Can you work these out from the drawing? Everything is in mm from the part's minimum corner. Coordinates: 2 decimals unless noted, no trailing zeros. Loops run counter-clockwise (first coordinate to the right, second up) from the corner with the lowest first, then second, coordinate; pieces in that order, holes last. Notation, with made-up numbers: (45.25, -37) - (78.25, -37) arc R14 ccw to (78.25, -30) - close; hole circle Ø10 at (36, -22.75). An arc over 180 degrees is marked (long way). Put each result on its own line as item: value. Start each with the question number.
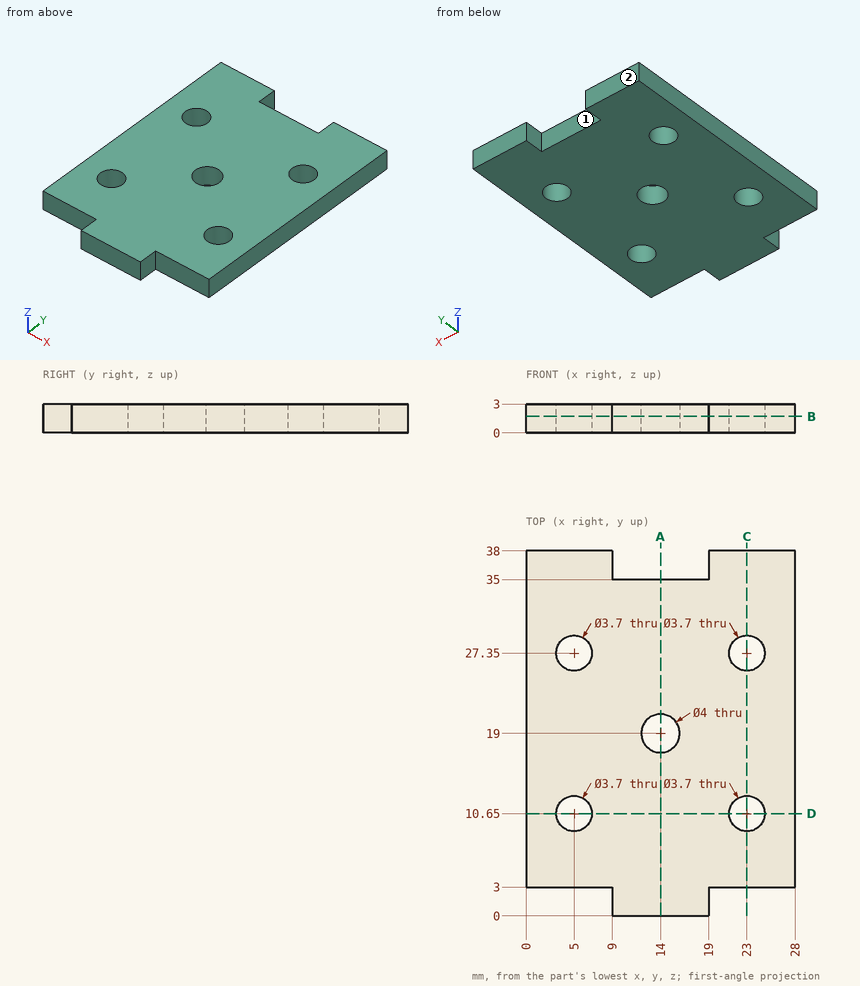
(1) I want a section at B-B on z = 1.7. List the corners of the cut face in (x, y) for me.
(2) I need wall thicknesses on L1, parallel to Y at x = 23, z = 1.85; L2, parallel to X at y = 9.5, z = 2.1; L3, parallel to Y at x = 22, z = 2.8. Which ranges of each line are inside material? Lowest first, please. Write a range as [from, to].
(3) For pin 1 Ø1.5 at (x, z) = (21.5, 1.5) entering from -Y; pin 2 Ø1.5 at (y, z) = (1.5, 1) entering from -X; pin 3 Ø0.9 at (x, z) = (15, 2) entering from +Y, each with a flat end and sliding along its axis, tell me the tip position at first contact or that it passes through.
(4) I want a section at C-C on x = 23. List the corners of the cut face in (y, z) for me.
(5) I want a section at A-A on x = 14. List the corners of the cut face in (y, z) for me, and give its area (3 significant figures).
(6) I want a section at D-D on y = 10.65. List the corners of the cut face in (x, z) for me.
(7) If we mould it in two halves opening along X, with no side actions, what happens to the marked faces 1 and 2? For each: pulls with the +X half, pulls with the -X half, needs draft (parallel to the pull), parting line crosses it, or undercut.
Answer sheet:
1. outline: (0, 3) - (9, 3) - (9, 0) - (19, 0) - (19, 3) - (28, 3) - (28, 38) - (19, 38) - (19, 35) - (9, 35) - (9, 38) - (0, 38) - close; hole circle Ø3.7 at (5, 10.65); hole circle Ø3.7 at (5, 27.35); hole circle Ø4 at (14, 19); hole circle Ø3.7 at (23, 10.65); hole circle Ø3.7 at (23, 27.35)
2. L1: y = [3, 8.8], [12.5, 25.5], [29.2, 38]
2. L2: x = [0, 3.55], [6.45, 21.55], [24.45, 28]
2. L3: y = [3, 9.09], [12.21, 25.79], [28.91, 38]
3. pin 1: stops at y = 3
3. pin 2: stops at x = 9
3. pin 3: stops at y = 35
4. outline: (3, 0) - (8.8, 0) - (8.8, 3) - (3, 3) - close; (12.5, 0) - (25.5, 0) - (25.5, 3) - (12.5, 3) - close; (29.2, 0) - (38, 0) - (38, 3) - (29.2, 3) - close
5. outline: (0, 0) - (17, 0) - (17, 3) - (0, 3) - close; (21, 0) - (35, 0) - (35, 3) - (21, 3) - close
5. area: 93.0 mm^2
6. outline: (0, 0) - (3.15, 0) - (3.15, 3) - (0, 3) - close; (6.85, 0) - (21.15, 0) - (21.15, 3) - (6.85, 3) - close; (24.85, 0) - (28, 0) - (28, 3) - (24.85, 3) - close
7. face 1: undercut
7. face 2: needs draft
